```python
from build123d import *

# Parameters (mm, degrees)
F1_DEPTH = 54.61
F3_DEPTH = 6.35


with BuildPart() as f1:
    # F0 (on Front) → F1 (new body)
    with BuildSketch(Plane.XZ):
        with BuildLine():
            Line((38.1, 0), (0, 0))
            Line((0, 0), (-38.1, 0))
            Line((-38.1, 0), (-59.436, -58.42))
            Line((-59.436, -58.42), (-51.816, -58.42))
            add(Edge.make_bspline(
                [(-51.816, -58.42), (-38.931578, -22.661388), (-18.689103, -20.525511), (0, -20.32)],
                knots=[0, 0, 0, 0, 64.315689, 64.315689, 64.315689, 64.315689], degree=3))
            add(Edge.make_bspline(
                [(51.816, -58.42), (38.931578, -22.661388), (18.689103, -20.525511), (0, -20.32)],
                knots=[0, 0, 0, 0, 64.315689, 64.315689, 64.315689, 64.315689], degree=3))
            Line((51.816, -58.42), (59.436, -58.42))
            Line((59.436, -58.42), (38.1, 0))
        make_face()
    extrude(amount=F1_DEPTH)

    # F2 (on face) → F3 (cut)
    with BuildSketch(Plane.XY):
        with BuildLine():
            Line((-19.431, -22.225), (19.431, -22.225))
            ThreePointArc((19.431, -22.225), (23.921128, -20.365128), (25.781, -15.875))
            Line((25.781, -15.875), (25.781, 0))
            Line((25.781, 0), (-25.781, 0))
            Line((-25.781, 0), (-25.781, -15.875))
            ThreePointArc((-25.781, -15.875), (-23.921128, -20.365128), (-19.431, -22.225))
        make_face()
        with BuildLine():
            Line((-25.781, -54.61), (25.781, -54.61))
            Line((25.781, -54.61), (25.781, -38.735))
            ThreePointArc((25.781, -38.735), (23.921128, -34.244872), (19.431, -32.385))
            Line((19.431, -32.385), (-19.431, -32.385))
            ThreePointArc((-19.431, -32.385), (-23.921128, -34.244872), (-25.781, -38.735))
            Line((-25.781, -38.735), (-25.781, -54.61))
        make_face()
    extrude(amount=-F3_DEPTH, mode=Mode.SUBTRACT)


solid = f1.part
```
Design review of the part built by this model. Coordinates are the model's own, in mm. A direction names the side the tool comes from. Coordinates: 2 decimals unless noted, no trailing zeros. Write each loop counter-clockwise with the first axis right and the second up, starting at its lowest first coordinate (ties: lowest second). Pieces come first, ordered by that corner, then holes.
1) Machinability: for faces 1 (the flat face through (-56, -27, -58.42)), 2 (the cylindrical face through (-23.871, -34.196, -3.131)), 3 (the cylindrical face through (23.871, -20.414, -3.131)), which of the approach directions +Z, -Z, +X, -X, +Y, -Y give a long, thin tool a straight path to every point of the face, cutting with its end or side? Answer none if there is none.
2) To check wall thickness, follow L1, parallel to X at y = -18.5, z = -27; L2, parallel to X at y = -29, z = -42; L3, parallel to Z at x = -16.5, y = -3.5. State the ranges of each line that lie inside material, in increasing order.
3) Insertion check: pin 1 (18 mm diameter, centred on x = 12, y = -48, fed in from +Z); pin 2 (3 mm diameter, centred on y = -45, z = -3.5, fed in from -X); pin 3 (1.5 mm diameter, centred on y = -16, z = -38.5, fed in from +X); pin 4 (12 mm diameter, centred on x = -4, z = -21, fed in from +Y). Each pin has a flat end and moves straight along its axis. Give the tip position at first contact, or say it passes through.
4) Add section A-A (z = -4). Write out the cut boundary in (x, y) (3 decimals), plus the area to 3 significant figures.
5) Add section C-C (z = -18.5). Write out the cut boundary in (x, y).
6) Add section B-B (z = -11). Write out the cut boundary in (x, y), plus the area to 3 significant figures.
7) Mouldability with a two-part tool opening along X and no side actions: class faces 4 (the flat face through (0, -54.61, -18)), 5 (the flat face through (25.781, -8, -3)), 6 (the flat face through (48.917, -26.923, -29.619)) as +X half, -X half, draft (parallel to the pull), parting line (faces both ways), or undercut.
Check result:
1. face 1: -Z, +X, -X, +Y, -Y
1. face 2: +Z, -Y
1. face 3: +Z, +Y
2. L1: x = -47.96 to -29.71, 29.71 to 47.96
2. L2: x = -53.44 to -44.08, 44.08 to 53.44
2. L3: z = -21.77 to -6.35
3. pin 1: stops at z = -6.35
3. pin 2: stops at x = -39.93
3. pin 3: stops at x = 52.43
3. pin 4: stops at y = 0
4. outline: (-39.561, -54.61) - (-25.781, -54.61) - (-25.781, -38.735) arc R6.35 cw to (-19.431, -32.385) - (19.431, -32.385) arc R6.35 cw to (25.781, -38.735) - (25.781, -54.61) - (39.561, -54.61) - (39.561, 0) - (25.781, 0) - (25.781, -15.875) arc R6.35 cw to (19.431, -22.225) - (-19.431, -22.225) arc R6.35 cw to (-25.781, -15.875) - (-25.781, 0) - (-39.561, 0) - close
4. area: 2,060 mm2
5. outline: (-44.86, -54.61) - (44.86, -54.61) - (44.86, 0) - (-44.86, 0) - close
6. outline: (-42.12, -54.61) - (42.12, -54.61) - (42.12, 0) - (-42.12, 0) - close
6. area: 4,600 mm2
7. face 4: draft
7. face 5: undercut
7. face 6: +X half
